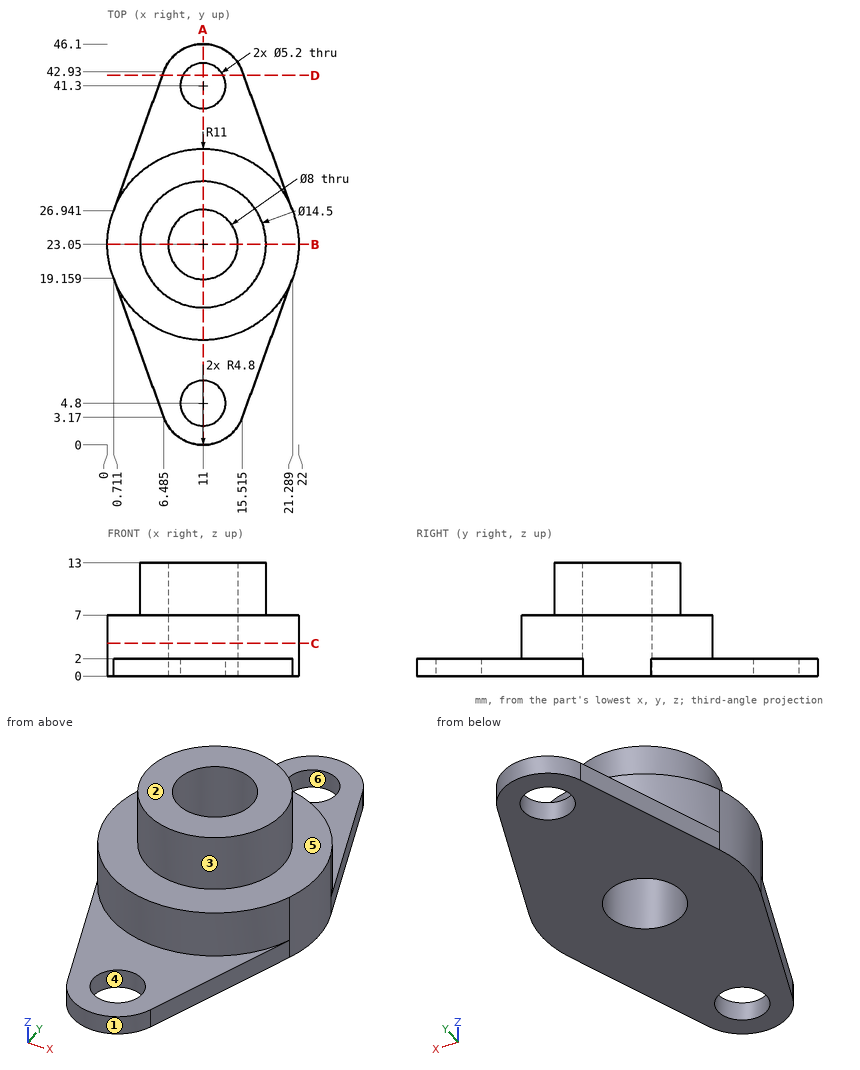
Geometry: see drawing. Coordinates: mm, zero at the bounding-box minimum. A direction names the side the tool comes from. Give positions to 0.01 mm unless a question says otherwise; leave off trailing zeros. Order: outer loops, then holes, each group sorted by start corner. A loop starts at its lowest first (then second) coordinate and runs counter-clockwise, first axis right, second up. Notation, with made-up numbers: (43.25, 83.25) -> (63.25, 83.25) arc R37 ccw to (63.25, 119.25) -> close; hole circle Ø3 at (26.25, -6.5). An arc over 180 degrees is marked (long way). Write each question's results on one line, items separated by ' | '.
1) Draft query along Y for the marked faces 1, 2, 3 and 4. Return one class per face: released by +Y, released by -Y, zero draft, split by the parting line, or undercut.
Geometry says:
face 1: released by -Y | face 2: zero draft | face 3: split by the parting line | face 4: undercut
2) Set-up query: the marked faces 5 and 6. Return all of +Z, -Z, +X, -X, +Y, -Y with unobstructed straight access to the full face (end or side cutting, diameter ignored); none if empty.
Geometry says:
face 5: +Z | face 6: +Z, -Z
3) Cut plane B-B (y = 23.05). Output: boundary loops of the cut face in (x, z), and give its area (3 significant figures).
Geometry says:
outline: (0, 0) -> (7, 0) -> (7, 13) -> (3.75, 13) -> (3.75, 7) -> (0, 7) -> close; (15, 0) -> (22, 0) -> (22, 7) -> (18.25, 7) -> (18.25, 13) -> (15, 13) -> close | area: 137 mm²
4) Cut plane A-A (x = 11). Output: boundary loops of the cut face in (y, z), and give its area (3 significant figures).
Geometry says:
outline: (0, 0) -> (2.2, 0) -> (2.2, 2) -> (0, 2) -> close; (7.4, 0) -> (19.05, 0) -> (19.05, 13) -> (15.8, 13) -> (15.8, 7) -> (12.05, 7) -> (12.05, 2) -> (7.4, 2) -> close; (27.05, 0) -> (38.7, 0) -> (38.7, 2) -> (34.05, 2) -> (34.05, 7) -> (30.3, 7) -> (30.3, 13) -> (27.05, 13) -> close; (43.9, 0) -> (46.1, 0) -> (46.1, 2) -> (43.9, 2) -> close | area: 164 mm²
5) First-contact query: pin 1 Ø12 at (x, y) = (16.5, 35.5) entering from +Z; pin 2 Ø2 at (y, z) = (19, 4) entering from +X; pin 3 Ø1 at (x, z) = (15, 8) entering from +Y. Flat tips, straight axial feed; report the tip coordinate or a pass-through.
Geometry says:
pin 1: stops at z = 7 | pin 2: stops at x = 21.57 | pin 3: stops at y = 29.4
6) Line query: line 1 along Y through (x, z) = (11, 0.5); line 2 along Y through (x, z) = (11, 9); line 3 along Y through (x, z) = (11, 4.25). Output: solid intervals per line, ascending.
Geometry says:
line 1: y = 0 to 2.2, 7.4 to 19.05, 27.05 to 38.7, 43.9 to 46.1 | line 2: y = 15.8 to 19.05, 27.05 to 30.3 | line 3: y = 12.05 to 19.05, 27.05 to 34.05
7) Cut plane D-D (y = 42.5). Output: boundary loops of the cut face in (x, z).
Geometry says:
outline: (6.33, 0) -> (8.69, 0) -> (8.69, 2) -> (6.33, 2) -> close; (13.31, 0) -> (15.67, 0) -> (15.67, 2) -> (13.31, 2) -> close
8) Cut plane C-C (z = 3.75). Output: boundary loops of the cut face in (x, y).
Geometry says:
outline: circle Ø22 at (11, 23.05); hole circle Ø8 at (11, 23.05)
